Part model, mm, in its own coordinate system. Coordinates: 2 decimals unless noted, no trailing zeros. Order: outer loops, then holes, each group sorted by start corner. A loop starts at its lowest first (then second) coordinate and runs counter-clockwise, first axis right, second up.
1) Cut at D-D (z = 5). List the corners of the cut face in (x, y), and give its area (3 significant figures).
2) Cut at C-C (z = 15). List the corners of the cut face in (x, y).
3) Cut at A-A (x = 1.35). List the corners of the cut face in (y, z), and give its area (3 significant figures).
4) Wall check: L1, parallel to Z at x = 5.05, y = 19.5; L2, parallel to Y at x = 3.8, z = 5; L3, parallel to Y at x = 0.55, z = 4. Give the ranges that are in metal, low to high.
5) Mould opens along Y. For faces 1 (the cylindrical face through (2.835, 12.834, 37.593)), 2 (the cylindrical face through (2.835, 5.56, 40.397)), 3 (the cylindrical face through (2.915, 64.804, 0.388)) say: +Y half, -Y half, draft (parallel to the pull), parting line (faces both ways), or undercut.
6) Cut at B-B (y = 12.5). List the corners of the cut face in (x, z), and give its area (3 significant figures).
7) Pin check, flat tip, straight feed: pin 1 Ø1.5 at (x, y) = (5, 11) entering from -Z. Stop position of the tip, or through.
```python
from build123d import *

# Parameters (mm, degrees)
SKETCH_1_R      = 7.6
SKETCH_1_R_2    = 2.1
SKETCH_1_R_3    = 2
EXTRUDE_1_DEPTH = 5.75
FILLET_1_R      = 5


with BuildPart() as part:
    # ｽｹｯﾁ1 → ﾎﾞｽ - 押し出し1 (new body)
    with BuildSketch(Plane(origin=(0, 0, 0), x_dir=(0, 0, -1), z_dir=(1, 0, 0))):
        with BuildLine():
            Line((-15, 0), (0, 15))
            Line((0, 15), (0, 65))
            Line((0, 65), (-11.532291921, 76.102082825))
            ThreePointArc((-11.532291921, 76.102082825), (-16.085919318, 77.380653566), (-19.667854572, 74.291963643))
            Line((-19.667854572, 74.291963643), (-41.669636429, 16.979909107))
            ThreePointArc((-41.669636429, 16.979909107), (-40.301671317, 5.420058752), (-30, 0))
            Line((-30, 0), (-15, 0))
        make_face()
        with Locations((-30, 12.5)):
            Circle(SKETCH_1_R, mode=Mode.SUBTRACT)
        with Locations((-5, 20)):
            Circle(SKETCH_1_R_2, mode=Mode.SUBTRACT)
        with Locations((-5, 60)):
            Circle(SKETCH_1_R_2, mode=Mode.SUBTRACT)
        with Locations((-15, 72.5)):
            Circle(SKETCH_1_R_3, mode=Mode.SUBTRACT)
    extrude(amount=EXTRUDE_1_DEPTH)

    # ﾌｨﾚｯﾄ1
    fillet_1_edges = [part.edges().sort_by_distance(p)[0] for p in [
        (2.875, 65, 0),
        (2.875, 15, 0),
        (2.875, 0, 15),
    ]]
    fillet(fillet_1_edges, radius=FILLET_1_R)


solid = part.part
```
Geometry check:
1. outline: (0, 10) - (5.75, 10) - (5.75, 17.9) - (0, 17.9) - close; (0, 22.1) - (5.75, 22.1) - (5.75, 57.9) - (0, 57.9) - close; (0, 62.1) - (5.75, 62.1) - (5.75, 69.81) - (0, 69.81) - close
1. area: 296 mm2
2. outline: (0, 0.45) - (5.75, 0.45) - (5.75, 70.5) - (0, 70.5) - close; (0, 74.5) - (5.75, 74.5) - (5.75, 77.5) - (0, 77.5) - close
3. outline: (0, 17.07) arc R5 ccw to (1.46, 13.54) - (13.54, 1.46) arc R5 ccw to (17.07, 0) - (62.87, 0) arc R5 ccw to (66.48, 1.53) - (76.1, 11.53) arc R5 ccw to (74.29, 19.67) - (16.98, 41.67) arc R12.5 ccw to (0, 30) - close; hole circle Ø15.2 at (12.5, 30); hole circle Ø4.2 at (20, 5); hole circle Ø4.2 at (60, 5); hole circle Ø4 at (72.5, 15)
3. area: 2,090 mm2
4. L1: z = 0 to 2.96, 7.04 to 27.04, 32.96 to 40.7
4. L2: y = 10 to 17.9, 22.1 to 57.9, 62.1 to 69.81
4. L3: y = 11 to 18.15, 21.85 to 58.15, 61.85 to 68.85
5. face 1: undercut
5. face 2: parting line
5. face 3: +Y half
6. outline: (0, 2.5) - (5.75, 2.5) - (5.75, 22.4) - (0, 22.4) - close; (0, 37.6) - (5.75, 37.6) - (5.75, 42.5) - (0, 42.5) - close
6. area: 143 mm2
7. pin 1: stops at z = 3.25
